Work out the finished part from the listing and answer in its coordinate system (mm). Coordinates: 2 decimals unless noted, no trailing zeros. Loops run counter-clockwise (first coordinate to the right, second up) from the corner with the lowest first, then second, coordinate; pieces in that order, holes last. Notation, with made-up numbers: (63, 73) -> (101, 73) arc R27 ccw to (101, 110) -> close; hole circle Ø10 at (52.5, 59.25). An arc over 180 degrees is marked (long way). Answer as CSV lines item,"result".
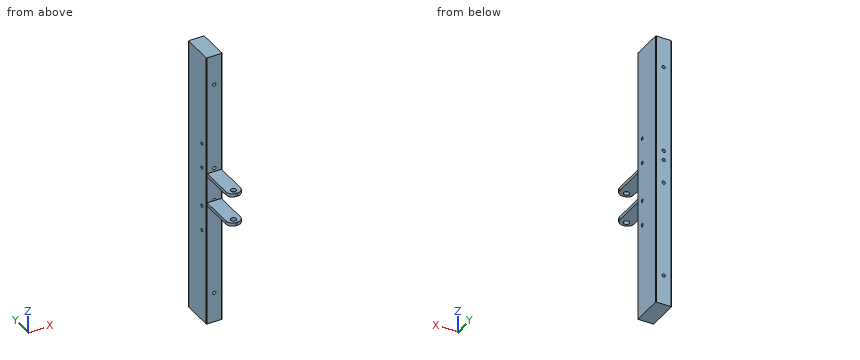
```python
from build123d import *

# Parameters (mm, degrees)
SKETCH_1_W          = 20
SKETCH_1_H          = 40
EXTRUDE_1_DEPTH     = 350
FILLET_1_R          = 1
SKETCH_2_R          = 2
CUT_EXTRUDE_1_DEPTH = 310
SKETCH_3_R          = 2
CUT_EXTRUDE_2_DEPTH = 90
SKETCH_4_W          = 18
SKETCH_4_H          = 4.110313015
EXTRUDE_2_DEPTH     = 50
SKETCH_5_R          = 3.525335322
CUT_EXTRUDE_3_DEPTH = 50
FILLET_2_R          = 8


with BuildPart() as part:
    # 草图1 → 凸台-拉伸1 (new body)
    with BuildSketch(Plane.XY):
        with Locations((10, 20)):
            Rectangle(SKETCH_1_W, SKETCH_1_H)
    extrude(amount=EXTRUDE_1_DEPTH)

    # 圆角1
    fillet_1_edges = [part.edges().sort_by_distance(p)[0] for p in [
        (0, 40, 175),
        (20, 40, 175),
        (20, 0, 175),
        (0, 0, 175),
    ]]
    fillet(fillet_1_edges, radius=FILLET_1_R)

    # 草图2 → 切除-拉伸1 (cut)
    with BuildSketch(Plane.ZY):
        with Locations((118, 10)):
            Circle(SKETCH_2_R)
        with Locations((232, 10)):
            Circle(SKETCH_2_R)
        with Locations((150, 10)):
            Circle(SKETCH_2_R)
        with Locations((200, 10)):
            Circle(SKETCH_2_R)
    extrude(amount=-CUT_EXTRUDE_1_DEPTH, mode=Mode.SUBTRACT)

    # 草图3 → 切除-拉伸2 (cut)
    with BuildSketch(Plane(origin=(0, 40, 0), x_dir=(1, 0, 0), z_dir=(0, 1, 0))):
        with Locations(Location((10, -38, 0), (0, 0, 270))):
            Circle(SKETCH_3_R)
        with Locations(Location((10, -312, 0), (0, 0, 270))):
            Circle(SKETCH_3_R)
        with Locations(Location((10, -160, 0), (0, 0, 270))):
            Circle(SKETCH_3_R)
        with Locations(Location((10, -190, 0), (0, 0, 270))):
            Circle(SKETCH_3_R)
        with Locations(Location((10, -202, 0), (0, 0, 270))):
            Circle(SKETCH_3_R)
    extrude(amount=-CUT_EXTRUDE_2_DEPTH, mode=Mode.SUBTRACT)

    # 草图4 → 凸台-拉伸2 (add)
    with BuildSketch(Plane.XZ):
        with Locations((10, 195.586566354)):
            Rectangle(SKETCH_4_W, SKETCH_4_H)
        with Locations((10, 157.223644883)):
            Rectangle(SKETCH_4_W, SKETCH_4_H)
    extrude(amount=EXTRUDE_2_DEPTH)

    # 草图5 → 切除-拉伸3 (cut)
    with BuildSketch(Plane(origin=(0, 0, 155.168488375), x_dir=(-1, 0, 0), z_dir=(0, 0, -1))):
        with Locations((-9.743882415, -43.170339686)):
            Circle(SKETCH_5_R)
    extrude(amount=-CUT_EXTRUDE_3_DEPTH, mode=Mode.SUBTRACT)

    # 圆角2
    fillet_2_edges = [part.edges().sort_by_distance(p)[0] for p in [
        (1, -50, 157.223644882),
        (19, -50, 157.223644882),
        (1, -50, 195.586566354),
        (19, -50, 195.586566354),
    ]]
    fillet(fillet_2_edges, radius=FILLET_2_R)


solid = part.part
```
(1) Flat-ended cylindrical pins translate along their axes: pin 1 Ø4.5 at (y, z) = (-27, 196.5) entering from +X; pin 2 Ø9 at (x, y) = (12, -13) entering from +Z; pin 3 Ø3.5 at (y, z) = (-14, 158) entering from -X; pin 4 Ø6.5 at (x, z) = (10, 38) entering from +Y. Find the tip coordinate at first contact, or state that the pin passes through.
Computed values:
pin 1,"x = 19"
pin 2,"z = 197.64"
pin 3,"x = 1"
pin 4,"y = 40"
(2) A cutting plane is placed at A-A, the plane y = -6. Write down the section's boundary in (x, z).
Computed values:
outline,"(1, 155.17) -> (19, 155.17) -> (19, 159.28) -> (1, 159.28) -> close; (1, 193.53) -> (19, 193.53) -> (19, 197.64) -> (1, 197.64) -> close"
(3) Consider line 1 along X through (y, z) = (17, 312); line 2 along Z through (x, y) = (10, -12.5); line 3 along Y through (x, z) = (4.5, 150). Determine where each line is inside the solid, lowest interval first.
Computed values:
line 1,"0 to 8, 12 to 20"
line 2,"155.17 to 159.28, 193.53 to 197.64"
line 3,"0 to 8, 12 to 40"
(4) A cutting plane is placed at B-B, the plane z = 285.5. Write down the section's boundary in (x, y).
Computed values:
outline,"(0, 1) arc R1 ccw to (1, 0) -> (19, 0) arc R1 ccw to (20, 1) -> (20, 39) arc R1 ccw to (19, 40) -> (1, 40) arc R1 ccw to (0, 39) -> close"
